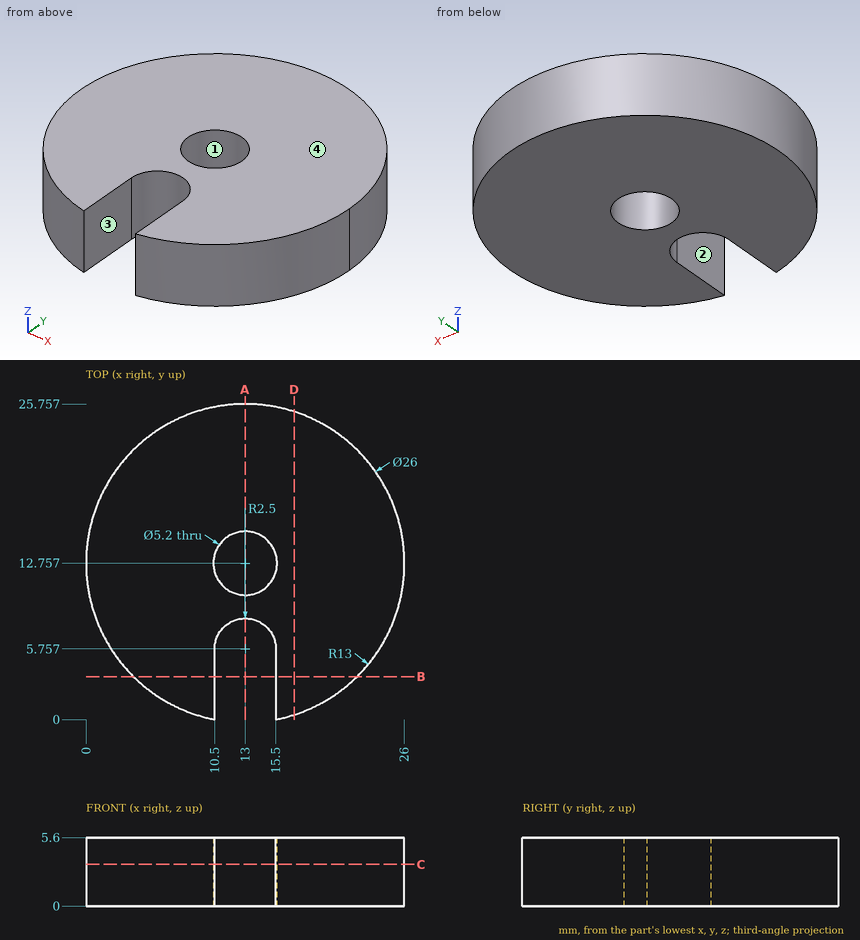
The drawing under review shows one solid part. Ordinate dimensions are in mm from its lowest x, y, z. A direction names the side the tool comes from. Round coordinates to 2 decimals unless told otherwise and drop trailing zeros. Write each loop counter-clockwise with the first axis right and the second up, starting at its lowest first coordinate (ties: lowest second). Pieces come first, ordered by that corner, then holes.
(1) Wall thickness on L1, parallel to Y at x = 13, z = 3.5; L2, parallel to X at y = 6, z = 4.9 (1 decimal); L3, parallel to Y at x = 11.75, z = 4.45: over which ranges is each line inside the solid? List them lowest first.
(2) We need section A-A on x = 13. Give the boundary of the cut face in (y, z).
(3) We need section B-B on y = 3.5. Give the boundary of the cut face in (x, z).
(4) We need section C-C on z = 3.4. Give the boundary of the cut face in (x, y), and give its area (3 significant figures).
(5) Machinability: for the marked faces 1 and 2, which of the approach directions +Z, -Z, +X, -X, +Y, -Y give a long, thin tool a straight path to every point of the face, cutting with its end or side? Answer none if there is none.
(6) We need section D-D on x = 17. Give the boundary of the cut face in (y, z).
(7) Mouldability with a two-part tool opening along X and no side actions: class the marked faces 3 and 4 as +X half, -X half, draft (parallel to the pull), parting line (faces both ways), or undercut.
(8) Insertion check: pin 1 (1 mm diameter, centred on y = 3, z = 2.5, fed in from -X); pin 2 (1.7 mm diameter, centred on y = 2, z = 2.5, fed in from +X); pin 3 (3 mm diameter, centred on y = 19.5, z = 4.5, fed in from -X). Each pin has a flat end and moves straight along its axis. Give the tip position at first contact, or say it passes through.
Findings below:
1. L1: y = 8.26 to 10.16, 15.36 to 25.76
1. L2: x = 1.9 to 10.5, 15.5 to 24.1
1. L3: y = 7.92 to 10.48, 15.04 to 25.7
2. outline: (8.26, 0) - (10.16, 0) - (10.16, 5.6) - (8.26, 5.6) - close; (15.36, 0) - (25.76, 0) - (25.76, 5.6) - (15.36, 5.6) - close
3. outline: (3.87, 0) - (10.5, 0) - (10.5, 5.6) - (3.87, 5.6) - close; (15.5, 0) - (22.13, 0) - (22.13, 5.6) - (15.5, 5.6) - close
4. outline: (10.5, 0) - (10.5, 5.76) arc R2.5 cw to (15.5, 5.76) - (15.5, 0) arc R13 ccw (long way) to start; hole circle Ø5.2 at (13, 12.76)
4. area: 470 mm2
5. face 1: +Z, -Z
5. face 2: +Z, -Z, -Y
6. outline: (0.39, 0) - (25.13, 0) - (25.13, 5.6) - (0.39, 5.6) - close
7. face 3: undercut
7. face 4: draft
8. pin 1: stops at x = 3.87
8. pin 2: stops at x = 21.42
8. pin 3: stops at x = 1.1
